Check sheet for the modelled part. Datum: model origin and axes. Units: mm. A direction names the side the tool comes from. Round coordinates to 2 decimals unless told otherwise and drop trailing zeros. Order: outer loops, then holes, each group sorted by start corner. A loop starts at its lowest first (then second) coordinate and runs counter-clockwise, first axis right, second up.
(1) Mould release check, pull along X, two halves, no side actions. Record for faces 6 (the flat face through (32, -33, 0)), 7 (the cylindrical face through (34.95, -21.83, 2.54)), 8 (the flat face through (62.83, -12.73, 2.46)): released by +X, released by -X, zero draft, split by the parting line, or undercut.
(2) Thickness scan on probe 1 along Y at (x, z) = (2, 2.4); probe 2 along Y at (x, z) = (71, 3.8); probe 3 along Y at (x, z) = (20, 3.9). Record the ranges inside material, lowest first.
(3) Sectioned sample at B-B, the plane x = 35. Enter the section's corners in (y, z).
(4) Tool access check on faces 1 (the flat face through (7.17, -47.27, 2.46)), 2 (the flat face through (54.7, -6.53, 2.46)), 3 (the cylindrical face through (45.366, -29.94, 2.535)), 4 (the flat face through (15.3, -53.47, 2.46)), 5 (the cylindrical face through (67.58, -58.144, 2.465)). Record the directions out of +Z, -Z, +X, -X, +Y, -Y that give a thin tool (end or side, any length) a straight path to the whole face; none if there is none.
(5) Sectioned sample at A-A, the plane z = 1.6. Enter the section's corners in (x, y), and give its area (3 significant figures).
(6) Sectioned sample at C-C, the plane y = -30. Enter the section's corners in (x, z).
Autodesk Inventor part; units mm, degrees
ref_plane "YZ Plane" through (0, 0, 0) normal (1, 0, 0) x (0, 1, 0)
ref_plane "XZ Plane" through (0, 0, 0) normal (0, 1, 0) x (-1, 0, 0)
ref_plane "XY Plane" through (0, 0, 0) normal (0, 0, 1) x (1, 0, 0)
sketch "Sketch1" plane through (0, 0, 0) normal (0, 0, 1) x (1, 0, 0)
  circle A0 centre (0, 0) radius 3
  circle A1 centre (0, -60) radius 3
  circle A2 centre (70, 0) radius 3
  circle A3 centre (70, -60) radius 3.05
  circle A4 centre (37.1599, -42) radius 6.15 construction
  line L0 (70, 0) -> (0, -60) construction
  line L1 (70, -60) -> (0, 0) construction
  circle A5 centre (35, -30) radius 2.5 construction
  line L2 (-1.607, 7.9628) -> (78.1149, -60.3703)
  line L3 (78.1149, -60.3703) -> (71.607, -67.9628)
  line L4 (71.607, -67.9628) -> (-8.1149, 0.3703)
  line L5 (-8.1149, 0.3703) -> (-1.607, 7.9628)
  line L6 (-1.607, 7.9628) -> (71.607, -67.9628) construction
  line L7 (78.1149, -60.3703) -> (-8.1149, 0.3703) construction
  line L8 (78.1149, 0.3703) -> (-1.607, -67.9628)
  line L9 (-1.607, -67.9628) -> (-8.1149, -60.3703)
  line L10 (-8.1149, -60.3703) -> (71.607, 7.9628)
  line L11 (71.607, 7.9628) -> (78.1149, 0.3703)
  line L12 (78.1149, 0.3703) -> (-8.1149, -60.3703) construction
  line L13 (-1.607, -67.9628) -> (71.607, 7.9628) construction
  point P0 (0, 0)
  dimension "d0" = 5
  dimension "d1" = 105
  dimension "d2" = 10
  dimension "d3" = 105
  dimension "d4" = 10
extrude "Extrusion1" add sketch "Sketch1" along normal blind 5
sketch "Sketch2" plane through (0, 0, 5) normal (0, 0, 1) x (1, 0, 0)
  circle A0 centre (0, -60) radius 3
  circle A1 centre (70, 0) radius 3
  circle A2 centre (70, -60) radius 3.05
  circle A3 centre (0, 0) radius 3
  line L0 (35, -23.4146) -> (-1.607, 7.9628)
  line L1 (-1.607, 7.9628) -> (-8.1149, 0.3703)
  line L2 (-8.1149, 0.3703) -> (27.317, -30)
  line L3 (27.317, -30) -> (-8.1149, -60.3703)
  line L4 (-8.1149, -60.3703) -> (-1.607, -67.9628)
  line L5 (-1.607, -67.9628) -> (35, -36.5854)
  line L6 (35, -36.5854) -> (71.607, -67.9628)
  line L7 (71.607, -67.9628) -> (78.1149, -60.3703)
  line L8 (78.1149, -60.3703) -> (42.683, -30)
  line L9 (42.683, -30) -> (78.1149, 0.3703)
  line L10 (78.1149, 0.3703) -> (71.607, 7.9628)
  line L11 (71.607, 7.9628) -> (35, -23.4146)
  circle A4 centre (35, -30) radius 3
  point P0 (0, 0)
  dimension "d7" = 6
extrude "Extrusion2" cut sketch "Sketch2" against normal through all contours A4
fillet "Fillet1" radius 5 4 edges at (35, -23.4146, 2.5) (27.317, -30, 2.5) (35, -36.5854, 2.5) (42.683, -30, 2.5)
properties part number "cellSTORM_inverted_LED"
Derived:
1. face 6: zero draft
1. face 7: undercut
1. face 8: released by +X
2. probe 1: y = -64.87 to -62.24, -57.76 to -51.7, -8.3 to -2.24, 2.24 to 4.87
2. probe 2: y = -67.44 to -62.88, -57.12 to -54.27, -5.73 to -2.83, 2.83 to 7.44
2. probe 3: y = -49.44 to -36.27, -23.73 to -10.56
3. outline: (-38.17, 0) - (-33, 0) - (-33, 5) - (-38.17, 5) - close; (-27, 0) - (-21.83, 0) - (-21.83, 5) - (-27, 5) - close
4. face 1: +Z, -Z, -X
4. face 2: +Z, -Z, +Y
4. face 3: +Z, -Z, +X
4. face 4: +Z, -Z, -Y
4. face 5: +Z, -Z
5. outline: (-8.11, -60.37) - (-1.61, -67.96) - (31.75, -39.37) arc R5 cw to (38.25, -39.37) - (71.61, -67.96) - (78.11, -60.37) - (47.11, -33.8) arc R5 cw to (47.11, -26.2) - (78.11, 0.37) - (71.61, 7.96) - (38.25, -20.63) arc R5 cw to (31.75, -20.63) - (-1.61, 7.96) - (-8.11, 0.37) - (22.89, -26.2) arc R5 cw to (22.89, -33.8) - close; hole circle Ø6 at (0, -60); hole circle Ø6 at (0, 0); hole circle Ø6 at (35, -30); hole circle Ø6.1 at (70, -60); hole circle Ø6 at (70, 0)
5. area: 1,880 mm2
6. outline: (24.63, 0) - (32, 0) - (32, 5) - (24.63, 5) - close; (38, 0) - (45.37, 0) - (45.37, 5) - (38, 5) - close
